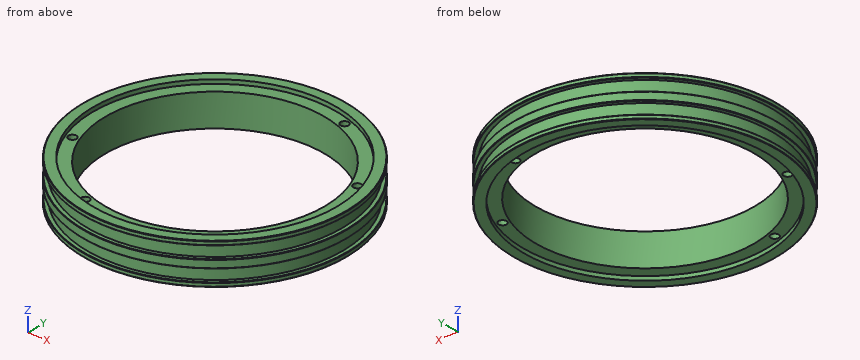
from build123d import *

# Parameters (mm, degrees)
SKETCH1_R           = 82.55
BOSS_EXTRUDE1_DEPTH = 25.4
SKETCH2_R           = 68.58
CUT_EXTRUDE1_DEPTH  = 25.4
SKETCH3_R           = 76.2
CUT_EXTRUDE2_DEPTH  = 2.54
CUT_EXTRUDE3_START  = -2.54
SKETCH4_R           = 76.2
CUT_EXTRUDE3_DEPTH  = 2.54
SKETCH5_W           = 2.54
SKETCH5_H           = 7.62
CHAMFER1_SIZE       = 0.254
CHAMFER2_SIZE       = 0.254
CHAMFER3_SIZE       = 0.254
CHAMFER4_SIZE       = 0.254
CHAMFER5_SIZE       = 0.254
CHAMFER6_SIZE       = 0.254
SKETCH6_R           = 2.54
CUT_EXTRUDE4_DEPTH  = 120.474537036


with BuildPart() as part:
    # Sketch1 → Boss-Extrude1 (new body)
    with BuildSketch(Plane.XY):
        Circle(SKETCH1_R)
    extrude(amount=BOSS_EXTRUDE1_DEPTH)

    # Sketch2 → Cut-Extrude1 (cut)
    with BuildSketch(Plane.XY):
        Circle(SKETCH2_R)
    extrude(amount=CUT_EXTRUDE1_DEPTH, mode=Mode.SUBTRACT)

    # Sketch3 → Cut-Extrude2 (cut)
    with BuildSketch(Plane.XY):
        Circle(SKETCH3_R)
    extrude(amount=CUT_EXTRUDE2_DEPTH, mode=Mode.SUBTRACT)

    # Sketch4 → Cut-Extrude3 (cut)
    with BuildSketch(Plane.XY.offset(25.4).offset(CUT_EXTRUDE3_START)):
        Circle(SKETCH4_R)
    extrude(amount=CUT_EXTRUDE3_DEPTH, mode=Mode.SUBTRACT)

    # Sketch5 → Cut-Revolve1 (revolve, cut)
    with BuildSketch(Plane(origin=(0, 0, 0), x_dir=(1, 0, 0), z_dir=(0, 1, 0))):
        with Locations((-81.28, -6.35)):
            Rectangle(SKETCH5_W, SKETCH5_H)
        with Locations((-81.28, -19.05)):
            Rectangle(SKETCH5_W, SKETCH5_H)
    revolve(axis=Axis((0, 0, 0), (0, 0, 1)), mode=Mode.SUBTRACT)

    # Chamfer1
    chamfer1_edges = [part.edges().sort_by_distance(p)[0] for p in [
        (-82.55, 0, 10.16),
    ]]
    chamfer(chamfer1_edges, length=CHAMFER1_SIZE)

    # Chamfer2
    chamfer2_edges = [part.edges().sort_by_distance(p)[0] for p in [
        (-82.55, 0, 15.24),
    ]]
    chamfer(chamfer2_edges, length=CHAMFER2_SIZE)

    # Chamfer3
    chamfer3_edges = [part.edges().sort_by_distance(p)[0] for p in [
        (-82.55, 0, 2.54),
    ]]
    chamfer(chamfer3_edges, length=CHAMFER3_SIZE)

    # Chamfer4
    chamfer4_edges = [part.edges().sort_by_distance(p)[0] for p in [
        (-82.55, 0, 22.86),
    ]]
    chamfer(chamfer4_edges, length=CHAMFER4_SIZE)

    # Chamfer5
    chamfer5_edges = [part.edges().sort_by_distance(p)[0] for p in [
        (-82.55, 0, 0),
    ]]
    chamfer(chamfer5_edges, length=CHAMFER5_SIZE)

    # Chamfer6
    chamfer6_edges = [part.edges().sort_by_distance(p)[0] for p in [
        (-82.55, 0, 25.4),
    ]]
    chamfer(chamfer6_edges, length=CHAMFER6_SIZE)

    # Sketch6 → Cut-Extrude4 (cut, through all)
    with BuildSketch(Plane.XY):
        with Locations((68.024348819, 24.758838175)):
            Circle(SKETCH6_R)
        with Locations((-68.024348819, -24.758838175)):
            Circle(SKETCH6_R)
        with Locations((24.758838175, 68.024348819)):
            Circle(SKETCH6_R)
        with Locations((-24.758838175, -68.024348819)):
            Circle(SKETCH6_R)
    extrude(amount=CUT_EXTRUDE4_DEPTH, mode=Mode.SUBTRACT)


solid = part.part
The listing builds one solid part. Answer for the finished solid, in the listing's coordinates (mm). Give positions to 0.01 mm unless a question says otherwise; leave off trailing zeros. Loops run counter-clockwise (first coordinate to the right, second up) from the corner with the lowest first, then second, coordinate; pieces in that order, holes last.
Item 1: A cutting plane is placed at B-B (x = -25). Give the number of separate pieces and of enclosed holes in the cut face, then the cut area to 3 significant figures.
Derived:
separate pieces: 3
enclosed holes: 0
area: 485 mm2
Item 2: A cutting plane is placed at A-A (z = 19.5). Give the vertices of the cut face in (x, y), then the cut area to 3 significant figures.
Derived:
outline: circle Ø160.02 at (0, 0); hole circle Ø5.08 at (-68.02, -24.76); hole circle Ø137.16 at (0, 0); hole circle Ø5.08 at (-24.76, -68.02); hole circle Ø5.08 at (24.76, 68.02); hole circle Ø5.08 at (68.02, 24.76)
area: 5,250 mm2
Item 3: Find the intervals of material crossed by line 1 along Y through (x, z) = (0, 1); line 2 along Y through (x, z) = (-23, 11.5); line 3 along X through (y, z) = (24, 11), in increasing order.
Derived:
line 1: y = -82.55 to -76.2, 76.2 to 82.55
line 2: y = -79.28 to -69.86, -66.19 to -64.61, 64.61 to 79.28
line 3: x = -78.98 to -64.24, 64.24 to 65.6, 70.45 to 78.98
Item 4: Each of these flat-tipped pins is pushed along its axis until it touches: pin 1 Ø2 at (x, z) = (38.5, 5.5) entering from -Y; pin 2 Ø8 at (x, y) = (68.02, 24.76) entering from -Z; pin 3 Ø6.5 at (x, y) = (-68.02, -24.76) entering from +Z; pin 4 Ø6 at (x, y) = (24.76, 68.02) entering from -Z. Where does it stop, or does it pass through?
Derived:
pin 1: stops at y = -70.68
pin 2: stops at z = 0
pin 3: stops at z = 22.86
pin 4: stops at z = 2.54
